Source: CAD feature listing. Evaluate the final solid. Frame: model axes, mm. Face numbers are marked on the shaded views. A direction names the side the tool comes from. Coordinates: 2 decimals unless noted, no trailing zeros. Order: outer loops, then holes, each group sorted by start corner. A loop starts at its lowest first (then second) coordinate and runs counter-clockwise, first axis right, second up.
Item 1: Section A-A on z = 22.5. Return the cut outline in (x, y).
Item 2: Section D-D on y = 30.5. Return the cut outline in (x, z), then the cut area to 3 significant figures.
Item 3: Reachability of the marked faces 4, 5, 6 and 7 from +Z, -Z, +X, -X, +Y, -Y: full face, straight path, thin tool, end or side. Return the list, or none.
Item 4: Mould query, pull axis X, two halves, no side actions, for the marked faces 1, 2 and 3. Classes: released by +X, released by -X, zero draft, split by the parting line, or undercut.
Item 5: Section C-C on x = 44. Return the cut outline in (y, z), then the cut area to 3 significant figures.
Item 6: Ray query, line 1 (X direction, y = 2.5, z = 22); line 2 (Y direction, x = 37, z = 11.5); line 3 (Z direction, x = 16, y = 14.5). Return the intervals inside material, ascending.
Item 7: Section B-B on y = 18.5. Return the cut outline in (x, z), then the cut area to 3 significant figures.
Item 8: Contact query for flat-ended pins moving along their axis: P1, Ø2, axis at x = 7, y = 5, coming from the +Z side; P2, Ø1.5, axis at x = 28.5, y = 7, coming from the -Z side; P3, Ø1.5, axis at y = 23.5, z = 13, coming from the +X side. Output: stop coordinate, or through.
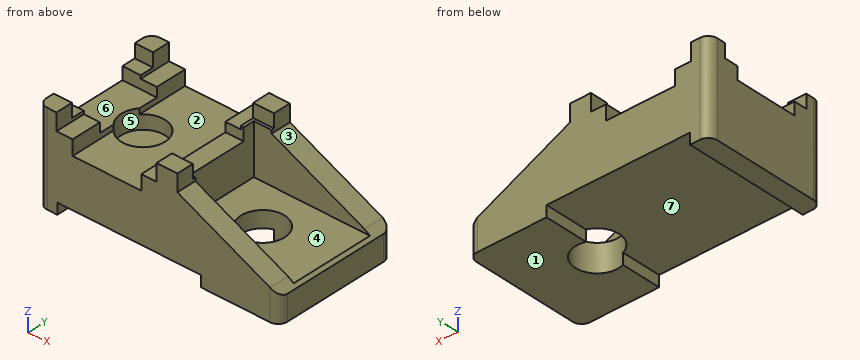
from build123d import *

# Parameters (mm, degrees)
F0_W      = 66.8964758515
F0_H      = 34.6800498664
F1_DEPTH  = 25.4
F2_R      = 6.0452
F3_DEPTH  = 25.401
F4_R      = 6.0753950253
F5_DEPTH  = 12.7
F6_W      = 33.2289449871
F6_H      = 23.5078325495
F6_R      = 6.0452
F7_DEPTH  = 17.78
F8_W      = 19.0628441051
F8_H      = 4.1393600404
F8_W_2    = 39.8685750552
F8_H_2    = 3.0596489087
F9_DEPTH  = 34.6810498664
F10_W     = 17.5169128925
F10_H     = 3.5316348076
F11_DEPTH = 66.8974758515
F12_R     = 2.54
F13_R     = 2.54
F15_DEPTH = 34.6810498664


with BuildPart() as f1:
    # F0 (on Top) → F1 (new body)
    with BuildSketch(Plane.XY):
        with Locations((33.4482379258, 17.3400249332)):
            Rectangle(F0_W, F0_H)
    extrude(amount=F1_DEPTH)

    # F2 (on face) → F3 (cut, through all)
    with BuildSketch(Plane.XY.offset(25.4)):
        with Locations((47.1864789724, 16.8195329607)):
            Circle(F2_R)
    extrude(amount=-F3_DEPTH, mode=Mode.SUBTRACT)

    # F4 (on face) → F5 (cut)
    with BuildSketch(Plane.XY.offset(25.4)):
        with Locations((14.1270142049, 16.6304875165)):
            Circle(F4_R)
    extrude(amount=-F5_DEPTH, mode=Mode.SUBTRACT)

    # F6 (on face) → F7 (cut)
    with BuildSketch(Plane.XY.offset(25.4)):
        with Locations((50.282003358, 17.2961675562)):
            Rectangle(F6_W, F6_H)
        with Locations((47.1864789724, 16.8195329607)):
            Circle(F6_R, mode=Mode.SUBTRACT)
    extrude(amount=-F7_DEPTH, mode=Mode.SUBTRACT)

    # F8 (on face) → F9 (cut, through all)
    with BuildSketch(Plane.XZ):
        with Locations((19.0694048069, 18.6367146671)):
            Rectangle(F8_W, F8_H)
        Polygon((32.8491181135, 25.4), (5.0718318671, 25.4), (5.0718318671, 20.7063946873), (9.5379827544, 20.7063946873), (28.6008268595, 20.7063946873), (32.8491181135, 20.7063946873), align=None)
        Polygon((66.8964758515, 25.4), (38.6224351823, 25.4), (66.8964758515, 6.9811479189), align=None)
        with Locations((25.2239794936, 1.5298244543)):
            Rectangle(F8_W_2, F8_H_2)
    extrude(amount=-F9_DEPTH, mode=Mode.SUBTRACT)

    # F10 (on face) → F11 (cut, through all)
    with BuildSketch(Plane(origin=(0, 0, 0), x_dir=(0, -1, 0), z_dir=(-1, 0, 0))):
        Polygon((-4.7551710159, 25.4), (-29.7591537237, 25.4), (-29.7591537237, 21.6030925512), (-25.944987312, 21.6030925512), (-8.4280744195, 21.6030925512), (-4.7551710159, 21.6030925512), align=None)
        with Locations((-17.1865308657, 19.8372751474)):
            Rectangle(F10_W, F10_H)
    extrude(amount=-F11_DEPTH, mode=Mode.SUBTRACT)

    # F12
    f12_edges = [f1.edges().sort_by_distance(p)[0] for p in [
        (66.896476, 0, 3.490574),
        (66.896476, 34.68005, 3.490574),
    ]]
    fillet(f12_edges, radius=F12_R)

    # F13
    f13_edges = [f1.edges().sort_by_distance(p)[0] for p in [
        (0, 34.68005, 12.7),
        (0, 0, 12.7),
    ]]
    fillet(f13_edges, radius=F13_R)

    # F14 (on face) → F15 (cut, through all)
    with BuildSketch(Plane.XZ):
        Polygon((64.3564758515, 8.6358065095), (38.6224351823, 25.4), (38.6224351823, 20.7063946873), align=None)
    extrude(amount=-F15_DEPTH, mode=Mode.SUBTRACT)


solid = f1.part
Answer list:
1. outline: (0, 2.54) arc R2.54 ccw to (2.54, 0) - (5.07, 0) - (5.07, 4.76) - (0, 4.76) - close; (0, 29.76) - (5.07, 29.76) - (5.07, 34.68) - (2.54, 34.68) arc R2.54 ccw to (0, 32.14) - close; (32.85, 0) - (38.62, 0) - (38.62, 4.76) - (32.85, 4.76) - close; (32.85, 29.76) - (38.62, 29.76) - (38.62, 34.68) - (32.85, 34.68) - close
2. outline: (0, 0) - (5.29, 0) - (5.29, 3.06) - (45.16, 3.06) - (45.16, 0) - (66.9, 0) - (66.9, 6.98) - (64.36, 8.64) - (38.62, 20.71) - (38.62, 25.4) - (32.85, 25.4) - (32.85, 20.71) - (28.6, 20.71) - (28.6, 16.57) - (9.54, 16.57) - (9.54, 20.71) - (5.07, 20.71) - (5.07, 25.4) - (0, 25.4) - close
2. area: 1,050 mm2
3. face 4: +Z, +X
3. face 5: +Z
3. face 6: +Z, +X, -X
3. face 7: -Z, +Y, -Y
4. face 1: zero draft
4. face 2: undercut
4. face 3: released by +X
5. outline: (0, 3.06) - (11.68, 3.06) - (11.68, 7.62) - (5.54, 7.62) - (5.54, 18.18) - (0, 18.18) - close; (21.96, 3.06) - (34.68, 3.06) - (34.68, 18.18) - (29.05, 18.18) - (29.05, 7.62) - (21.96, 7.62) - close
5. area: 229 mm2
6. line 1: x = 0 to 5.07, 32.85 to 38.62
6. line 2: y = 0 to 5.54, 29.05 to 34.68
6. line 3: z = 3.06 to 12.7
7. outline: (0, 0) - (5.29, 0) - (5.29, 3.06) - (41.38, 3.06) - (41.38, 7.62) - (33.67, 7.62) - (33.67, 18.07) - (28.6, 18.07) - (28.6, 16.57) - (19.91, 16.57) - (19.91, 12.7) - (8.35, 12.7) - (8.35, 18.07) - (0, 18.07) - close; (52.99, 0) - (66.9, 0) - (66.9, 6.98) - (65.92, 7.62) - (52.99, 7.62) - close
7. area: 587 mm2
8. P1: stops at z = 20.71
8. P2: stops at z = 3.06
8. P3: stops at x = 33.67
